Part model, mm, in its own coordinate system. Give positions to 0.01 mm unless a question says otherwise; leave off trailing zeros. Loops run counter-clockwise (first coordinate to the right, second up) from the corner with the lowest first, then second, coordinate; pieces in that order, holes last. Notation, with made-up numbers: M 47,53.25 L 52,53.25 A30 cw 52,78.25 Z; hole C 19,57 d4. An arc over 180 degrees is marked long. Answer in a Markdown table with one row per item.
from build123d import *

# Parameters (mm, degrees)
SKETCH1_W           = 38.5
SKETCH1_H           = 62
BOSS_EXTRUDE1_DEPTH = 8.5
FILLET1_R           = 3
SKETCH2_R           = 0.325
BOSS_EXTRUDE2_DEPTH = 8.5


with BuildPart() as part:
    # Sketch1 → Boss-Extrude1 (new body)
    with BuildSketch(Plane(origin=(0, 0, 0), x_dir=(1, 0, 0), z_dir=(0, 1, 0))):
        Rectangle(SKETCH1_W, SKETCH1_H)
    extrude(amount=BOSS_EXTRUDE1_DEPTH)

    # Fillet1
    fillet1_edges = [part.edges().sort_by_distance(p)[0] for p in [
        (-19.25, 8.5, 0),
        (19.25, 8.5, 0),
        (-19.25, 0, 0),
        (19.25, 0, 0),
    ]]
    fillet(fillet1_edges, radius=FILLET1_R)

    # Sketch2 → Boss-Extrude2 (add)
    with BuildSketch(Plane.XY.offset(31)):
        with Locations(Location((-1, 4.25, 0), (0, 0, 180))):
            Circle(SKETCH2_R)
        with Locations(Location((1, 4.25, 0), (0, 0, 180))):
            Circle(SKETCH2_R)
    extrude(amount=BOSS_EXTRUDE2_DEPTH)


solid = part.part
(1) Drill centre lines: line 1 along Z through (x, y) = (-6, 8); line 2 along X through (y, z) = (8, -12.5); line 3 along X through (y, z) = (2.5, -21.5). Where is each one in solid material? Low to high.
Recorded:
| item | result |
|---|---|
| line 1 | z = -31 to 31 |
| line 2 | x = -17.91 to 17.91 |
| line 3 | x = -19.21 to 19.21 |
(2) Saw through at A-A (z = 3.5). Write the cut outline in (x, y).
Recorded:
| item | result |
|---|---|
| outline | M -19.25,3 A3 ccw -16.25,0 L 16.25,0 A3 ccw 19.25,3 L 19.25,5.5 A3 ccw 16.25,8.5 L -16.25,8.5 A3 ccw -19.25,5.5 Z |
(3) Saw through at C-C (y = 2.25). Write the cut outline in (x, z).
Recorded:
| item | result |
|---|---|
| outline | M -19.15,-31 L 19.15,-31 L 19.15,31 L -19.15,31 Z |
(4) Saw through at B-B (x = -10.5). Write the cut outline in (y, z).
Recorded:
| item | result |
|---|---|
| outline | M 0,-31 L 8.5,-31 L 8.5,31 L 0,31 Z |
(5) Pin check, flat tips, straight feed: pin 1 Ø5 at (y, z) = (2.5, 24) entering from -X; pin 2 Ø5 at (x, y) = (5.5, 6) entering from +Z. Stop position of each tip, or through.
Recorded:
| item | result |
|---|---|
| pin 1 | stops at x = -19.25 |
| pin 2 | stops at z = 31 |
